Build history of the part. All positions in model axes, mm. Face numbers are marked on the shaded views. A direction names the side the tool comes from. Coordinates: 2 decimals unless noted, no trailing zeros. Loops run counter-clockwise (first coordinate to the right, second up) from the corner with the lowest first, then second, coordinate; pieces in that order, holes last.
(1) Slice it at D-D (y = 26). Give the cut face in (x, z), and give its area (3 significant figures).
(2) Wall check: L1, parallel to Y at x = 27.3, z = 8.5; L2, parallel to Y at x = 34, z = 25; L3, parallel to Y at x = 33.5, z = 10.5. Give the ranges that are in metal, low to high.
(3) Flat gauge pins, fed straight in: P1, Ø5, axis at x = 22.5, y = 15, coming from the +Z side; P2, Ø1, axis at x = 30, y = 16, coming from the -Z side; P3, Ø5, axis at y = 7, z = 4, coming from the -X side; P4, Ø4, axis at x = 45.7, z = 11.32, coming from the -Y side. Where does each tip first touch, or does it go through?
(4) Slice it at B-B (y = 2.5). Give the cut face in (x, z), and give its area (3 significant figures).
(5) Slice it at C-C (x = 25). Give the cut face in (y, z), and give its area (3 significant figures).
(6) Tool access for the marked faces 5, 6, 7 and 8: list every direction of +Z, -Z, +X, -X, +Y, -Y with a clear straight run to the whole face (end or side of a thin tool).
(7) Slice it at A-A (z = 17). Give the cut face in (x, y).
(8) Two-plate mould, pull along X, no slides. Class the marked faces 1, 2, 3 and 4: pulls with the +X half, pulls with the -X half, needs draft (parallel to the pull), parting line crosses it, or undercut.
from build123d import *

# Parameters (mm, degrees)
RESSALTO_EXTRUS_O1_DEPTH    = 30
CORTE_EXTRUS_O1_DEPTH       = 54.488316481
CORTE_EXTRUS_O1_DEPTH_BACK  = 54.488316481
ESBO_O3_R                   = 1.1
CORTE_EXTRUS_O6_DEPTH       = 54.488316481
CORTE_EXTRUS_O6_DEPTH_BACK  = 54.488316481
ESBO_O4_W                   = 12
ESBO_O4_H                   = 15
ESBO_O5_R                   = 1.6
CORTE_EXTRUS_O7_DEPTH       = 54.488316481
CORTE_EXTRUS_O9_START       = 6
ESBO_O7_W                   = 15
ESBO_O7_H                   = 15
CORTE_EXTRUS_O9_DEPTH       = 8
CORTE_EXTRUS_O11_REACH      = 55.488
ESBO_O9_R                   = 1.6
ESBO_O8_R                   = 3
CORTE_EXTRUS_O10_DEPTH      = 2
CORTE_EXTRUS_O14_DEPTH      = 43.308391603
CORTE_EXTRUS_O14_DEPTH_BACK = 2
CORTE_EXTRUS_O16_DEPTH      = 55.626001135
CORTE_EXTRUS_O16_DEPTH_BACK = 1
ESBO_O15_R                  = 2.1
FILETE1_R                   = 4
ESBO_O16_W                  = 10
ESBO_O16_H                  = 3.82
RESSALTO_EXTRUS_O2_DEPTH    = 2
ESBO_O17_W                  = 15.9
ESBO_O17_H                  = 2.8
RESSALTO_EXTRUS_O3_DEPTH    = 3.5
ESBO_O18_W                  = 52.248887689
ESBO_O18_H                  = 54.313207189
CORTE_EXTRUS_O17_DEPTH      = 34
ESBO_O19_R                  = 3.6
ESBO_O19_R_2                = 1.6
RESSALTO_EXTRUS_O4_DEPTH    = 6


with BuildPart() as part:
    # Esboço1 → Ressalto-extrusão1 (new body)
    with BuildSketch(Plane.XY):
        with BuildLine():
            Line((0, 0), (3, 0))
            Line((3, 0), (3, 8))
            ThreePointArc((3, 8), (4.464466094, 11.535533906), (8, 13))
            Line((8, 13), (15, 13))
            Line((15, 13), (15, 21))
            Line((15, 21), (-13, 21))
            Line((-13, 21), (-13, 36))
            Line((-13, 36), (1, 36))
            Line((1, 36), (1, 40))
            Line((1, 40), (-19, 40))
            Line((-19, 40), (-19, 17))
            Line((-19, 17), (0, 17))
            Line((0, 17), (0, 0))
        make_face()
    extrude(amount=RESSALTO_EXTRUS_O1_DEPTH)

    # Esboço3 → Corte-extrusão1 (cut, two sides: drawn at the far end of the back side and taken through both)
    with BuildSketch(Plane(origin=(0, 0, 0), x_dir=(0, 0, -1), z_dir=(1, 0, 0)).offset(-CORTE_EXTRUS_O1_DEPTH_BACK)):
        with Locations((-8.5, 14.5)):
            Circle(ESBO_O3_R)
        with Locations(Location((-21.5, 14.5, 0), (0, 0, 90))):
            Circle(ESBO_O3_R)
        with Locations(Location((-8.5, 2.5, 0), (0, 0, 90))):
            Circle(ESBO_O3_R)
        with Locations(Location((-21.5, 2.5, 0), (0, 0, 90))):
            Circle(ESBO_O3_R)
    extrude(amount=CORTE_EXTRUS_O1_DEPTH + CORTE_EXTRUS_O1_DEPTH_BACK, mode=Mode.SUBTRACT)

    # Esboço4 → Corte-extrusão6 (cut, two sides: drawn at the far end of the back side and taken through both)
    with BuildSketch(Plane(origin=(0, 0, 0), x_dir=(1, 0, 0), z_dir=(0, 1, 0)).offset(-CORTE_EXTRUS_O6_DEPTH_BACK)):
        with Locations((9, -22.5)):
            Rectangle(ESBO_O4_W, ESBO_O4_H)
    extrude(amount=CORTE_EXTRUS_O6_DEPTH + CORTE_EXTRUS_O6_DEPTH_BACK, mode=Mode.SUBTRACT)

    # Esboço5 → Corte-extrusão7 (cut, through all)
    with BuildSketch(Plane(origin=(0, 40, 0), x_dir=(1, 0, 0), z_dir=(0, 1, 0))):
        with Locations(Location((-5, -22, 0), (0, 0, 270))):
            Circle(ESBO_O5_R)
        with Locations(Location((-15.7, -11.32, 0), (0, 0, 180))):
            Circle(ESBO_O5_R)
        with Locations(Location((11, -7.5, 0), (0, 0, 180))):
            Circle(ESBO_O5_R)
    extrude(amount=-CORTE_EXTRUS_O7_DEPTH, mode=Mode.SUBTRACT)

    # Esboço7 → Corte-extrusão9 (cut)
    with BuildSketch(Plane(origin=(0, 21, 0), x_dir=(1, 0, 0), z_dir=(0, 1, 0)).offset(CORTE_EXTRUS_O9_START)):
        with Locations((-15.7, -11.32)):
            Rectangle(ESBO_O7_W, ESBO_O7_H)
    extrude(amount=CORTE_EXTRUS_O9_DEPTH, mode=Mode.SUBTRACT)

    # Esboço9 → Corte-extrusão11 (cut, up to next)
    with BuildSketch(Plane(origin=(0, 40, 0), x_dir=(1, 0, 0), z_dir=(0, 1, 0)), mode=Mode.PRIVATE) as corte_extrus_o11_sk1:
        with Locations(Location((-4, -7.5, 0), (0, 0, 180))):
            Circle(ESBO_O9_R)
    corte_extrus_o11_tool1 = extrude(corte_extrus_o11_sk1.sketch, amount=-CORTE_EXTRUS_O11_REACH, mode=Mode.PRIVATE) & part.part
    add(corte_extrus_o11_tool1.solids().sort_by_distance((-4, 40, 7.5))[0], mode=Mode.SUBTRACT)

    # Esboço8 → Corte-extrusão10 (cut)
    with BuildSketch(Plane(origin=(0, 40, 0), x_dir=(1, 0, 0), z_dir=(0, 1, 0))):
        with Locations(Location((-15.7, -11.32, 0), (0, 0, 180))):
            Circle(ESBO_O8_R)
        with Locations(Location((-5, -22, 0), (0, 0, 180))):
            Circle(ESBO_O8_R)
        with Locations(Location((-4, -7.5, 0), (0, 0, 180))):
            Circle(ESBO_O8_R)
    extrude(amount=-CORTE_EXTRUS_O10_DEPTH, mode=Mode.SUBTRACT)

    # Esboço14 → Corte-extrusão14 (cut, two sides: drawn at the far end of the back side and taken through both)
    with BuildSketch(Plane.XZ.offset(-17).offset(-CORTE_EXTRUS_O14_DEPTH_BACK)):
        with BuildLine():
            Line((11, 11), (15, 11))
            Line((15, 11), (15, 4))
            Line((15, 4), (11, 4))
            ThreePointArc((11, 4), (7.5, 7.5), (11, 11))
        make_face()
        Polygon((-5, 25.233161507), (-7.8, 23.616580754), (-7.8, 20.383419246), (-5, 18.766838493), (-2.2, 20.383419246), (-2.2, 23.616580754), align=None)
        Polygon((-15.7, 14.553161507), (-18.5, 12.936580754), (-18.5, 9.703419246), (-15.7, 8.086838493), (-12.9, 9.703419246), (-12.9, 12.936580754), align=None)
    extrude(amount=CORTE_EXTRUS_O14_DEPTH + CORTE_EXTRUS_O14_DEPTH_BACK, mode=Mode.SUBTRACT)

    # Esboço15 → Corte-extrusão16 (cut, two sides: drawn at the far end of the back side and taken through both)
    with BuildSketch(Plane(origin=(3, 0, 0), x_dir=(0, 0, -1), z_dir=(1, 0, 0)).offset(-CORTE_EXTRUS_O16_DEPTH_BACK)):
        with Locations(Location((-21.5, 14.5, 0), (0, 0, 90))):
            Circle(ESBO_O15_R)
        with Locations(Location((-8.5, 14.5, 0), (0, 0, 313.540252108))):
            Circle(ESBO_O15_R)
        with Locations(Location((-8.5, 2.5, 0), (0, 0, 90))):
            Circle(ESBO_O15_R)
        with Locations(Location((-21.5, 2.5, 0), (0, 0, 90))):
            Circle(ESBO_O15_R)
    extrude(amount=CORTE_EXTRUS_O16_DEPTH + CORTE_EXTRUS_O16_DEPTH_BACK, mode=Mode.SUBTRACT)

    # Filete1
    # the kernel refuses this fillet: 4 mm, written as the material it adds along each edge
    with BuildSketch(Plane(origin=(-13, 21, 0), x_dir=(1, 0, 0), z_dir=(0, 0, 1))) as filete1_piece_1:
        with BuildLine():
            CenterArc((FILETE1_R, FILETE1_R), FILETE1_R, 180, 90)
            Line((0, FILETE1_R), (0, 0))
            Line((0, 0), (FILETE1_R, 0))
        make_face()
    extrude(amount=30)
    with BuildSketch(Plane(origin=(-13, 36, 0), x_dir=(1, 0, 0), z_dir=(0, 0, 1))) as filete1_piece_2_section:
        with BuildLine():
            CenterArc((FILETE1_R, -FILETE1_R), FILETE1_R, 90, 90)
            Line((0, -FILETE1_R), (0, 0))
            Line((0, 0), (FILETE1_R, 0))
        make_face()
    filete1_piece_2 = extrude(amount=30, mode=Mode.PRIVATE)
    filete1_piece_2 = split(filete1_piece_2, bisect_by=Plane(origin=(-11.759467995, 35, 1.91), z_dir=(0, 1, 0)), keep=Keep.TOP, mode=Mode.PRIVATE)
    filete1_piece_2 = split(filete1_piece_2, bisect_by=Plane(origin=(-11.759467995, 35.634662641, 3.82), z_dir=(0, 0, -1)), keep=Keep.TOP, mode=Mode.PRIVATE)
    add(filete1_piece_2)
    with BuildSketch(Plane(origin=(-13, 36, 0), x_dir=(1, 0, 0), z_dir=(0, 0, 1))) as filete1_piece_3_section:
        with BuildLine():
            CenterArc((FILETE1_R, -FILETE1_R), FILETE1_R, 90, 90)
            Line((0, -FILETE1_R), (0, 0))
            Line((0, 0), (FILETE1_R, 0))
        make_face()
    filete1_piece_3 = extrude(amount=30, mode=Mode.PRIVATE)
    filete1_piece_3 = split(filete1_piece_3, bisect_by=Plane(origin=(-12.678584174, 35, 1.91), z_dir=(0, -1, 0)), keep=Keep.TOP, mode=Mode.PRIVATE)
    filete1_piece_3 = split(filete1_piece_3, bisect_by=Plane(origin=(-12.678584174, 34.15222085, 3.82), z_dir=(0, 0, -1)), keep=Keep.TOP, mode=Mode.PRIVATE)
    add(filete1_piece_3)
    with BuildSketch(Plane(origin=(-13, 36, 0), x_dir=(1, 0, 0), z_dir=(0, 0, 1))) as filete1_piece_4_section:
        with BuildLine():
            CenterArc((FILETE1_R, -FILETE1_R), FILETE1_R, 90, 90)
            Line((0, -FILETE1_R), (0, 0))
            Line((0, 0), (FILETE1_R, 0))
        make_face()
    filete1_piece_4 = extrude(amount=30, mode=Mode.PRIVATE)
    filete1_piece_4 = split(filete1_piece_4, bisect_by=Plane(origin=(-11.759467995, 35, 11.32), z_dir=(0, 1, 0)), keep=Keep.TOP, mode=Mode.PRIVATE)
    filete1_piece_4 = split(filete1_piece_4, bisect_by=Plane(origin=(-11.759467995, 35.634662641, 3.82), z_dir=(0, 0, 1)), keep=Keep.TOP, mode=Mode.PRIVATE)
    filete1_piece_4 = split(filete1_piece_4, bisect_by=Plane(origin=(-11.759467995, 35.634662641, 18.82), z_dir=(0, 0, -1)), keep=Keep.TOP, mode=Mode.PRIVATE)
    add(filete1_piece_4)
    with BuildSketch(Plane(origin=(-13, 36, 0), x_dir=(1, 0, 0), z_dir=(0, 0, 1))) as filete1_piece_5_section:
        with BuildLine():
            CenterArc((FILETE1_R, -FILETE1_R), FILETE1_R, 90, 90)
            Line((0, -FILETE1_R), (0, 0))
            Line((0, 0), (FILETE1_R, 0))
        make_face()
    filete1_piece_5 = extrude(amount=30, mode=Mode.PRIVATE)
    filete1_piece_5 = split(filete1_piece_5, bisect_by=Plane(origin=(-11.759467995, 35, 24.41), z_dir=(0, 1, 0)), keep=Keep.TOP, mode=Mode.PRIVATE)
    filete1_piece_5 = split(filete1_piece_5, bisect_by=Plane(origin=(-11.759467995, 35.634662641, 18.82), z_dir=(0, 0, 1)), keep=Keep.TOP, mode=Mode.PRIVATE)
    add(filete1_piece_5)
    with BuildSketch(Plane(origin=(-13, 36, 0), x_dir=(1, 0, 0), z_dir=(0, 0, 1))) as filete1_piece_6_section:
        with BuildLine():
            CenterArc((FILETE1_R, -FILETE1_R), FILETE1_R, 90, 90)
            Line((0, -FILETE1_R), (0, 0))
            Line((0, 0), (FILETE1_R, 0))
        make_face()
    filete1_piece_6 = extrude(amount=30, mode=Mode.PRIVATE)
    filete1_piece_6 = split(filete1_piece_6, bisect_by=Plane(origin=(-12.678584174, 35, 24.41), z_dir=(0, -1, 0)), keep=Keep.TOP, mode=Mode.PRIVATE)
    filete1_piece_6 = split(filete1_piece_6, bisect_by=Plane(origin=(-12.678584174, 34.15222085, 18.82), z_dir=(0, 0, 1)), keep=Keep.TOP, mode=Mode.PRIVATE)
    add(filete1_piece_6)
    # the kernel refuses this fillet: 4 mm, written as the material it takes off along each edge
    with BuildSketch(Plane(origin=(-10, 0, 0), x_dir=(0, 0, 1), z_dir=(1, 0, 0))) as filete1_2_piece_1:
        with BuildLine():
            CenterArc((FILETE1_R, -FILETE1_R), FILETE1_R, 90, 90)
            Line((0, -FILETE1_R), (0, 0))
            Line((0, 0), (FILETE1_R, 0))
        make_face()
    extrude(amount=23, mode=Mode.SUBTRACT)
    with BuildSketch(Plane(origin=(-10, 0, 30), x_dir=(0, 0, -1), z_dir=(1, 0, 0))) as filete1_2_piece_2:
        with BuildLine():
            CenterArc((FILETE1_R, FILETE1_R), FILETE1_R, 180, 90)
            Line((0, FILETE1_R), (0, 0))
            Line((0, 0), (FILETE1_R, 0))
        make_face()
    extrude(amount=23, mode=Mode.SUBTRACT)
    with BuildSketch(Plane(origin=(3, 21, 15), x_dir=(-1, 0, 0), z_dir=(0, 0, 1))) as filete1_2_piece_3:
        with BuildLine():
            CenterArc((FILETE1_R, FILETE1_R), FILETE1_R, 180, 90)
            Line((0, FILETE1_R), (0, 0))
            Line((0, 0), (FILETE1_R, 0))
        make_face()
    extrude(amount=25, mode=Mode.SUBTRACT)
    with BuildSketch(Plane(origin=(1, 26, 0), x_dir=(0, 0, 1), z_dir=(0, 1, 0)), Plane(origin=(15, 13, -10), x_dir=(-1, 0, 0), z_dir=(0, 0, 1)), Plane(origin=(15, 13, 1), x_dir=(-1, 0, 0), z_dir=(0, 0, 1))) as filete1_2_piece_4:
        with BuildLine():
            CenterArc((FILETE1_R, -FILETE1_R), FILETE1_R, 90, 90)
            Line((0, -FILETE1_R), (0, 0))
            Line((0, 0), (FILETE1_R, 0))
        make_face()
    extrude(amount=24, mode=Mode.SUBTRACT)
    with BuildSketch(Plane(origin=(1, 26, 30), x_dir=(0, 0, -1), z_dir=(0, 1, 0))) as filete1_2_piece_5:
        with BuildLine():
            CenterArc((FILETE1_R, FILETE1_R), FILETE1_R, 180, 90)
            Line((0, FILETE1_R), (0, 0))
            Line((0, 0), (FILETE1_R, 0))
        make_face()
    extrude(amount=24, mode=Mode.SUBTRACT)

    # Esboço16 → Ressalto-extrusão2 (add)
    with BuildSketch(Plane(origin=(0, 21, 0), x_dir=(1, 0, 0), z_dir=(0, 1, 0))):
        with Locations((-14, -1.91)):
            Rectangle(ESBO_O16_W, ESBO_O16_H)
    extrude(amount=RESSALTO_EXTRUS_O2_DEPTH)

    # Esboço17 → Ressalto-extrusão3 (add)
    with BuildSketch(Plane(origin=(0, 21, 0), x_dir=(1, 0, 0), z_dir=(0, 1, 0))):
        with Locations((-1.05, -7.5)):
            Rectangle(ESBO_O17_W, ESBO_O17_H)
    extrude(amount=RESSALTO_EXTRUS_O3_DEPTH)

    # Espelhar1: part across plane


with BuildPart() as part_1:
    add(part.part)
    add(part.part.mirror(Plane(origin=(15, 21, 30), x_dir=(0, 0, 1), z_dir=(-1, 0, 0))))

    # Esboço18 → Corte-extrusão17 (cut)
    with BuildSketch(Plane.ZY.offset(19)):
        with Locations((14.699236255, 19.293263453)):
            Rectangle(ESBO_O18_W, ESBO_O18_H)
    extrude(amount=-CORTE_EXTRUS_O17_DEPTH, mode=Mode.SUBTRACT)

    # Esboço19 → Ressalto-extrusão4 (add)
    with BuildSketch(Plane.XZ.offset(-36)):
        with Locations(Location((35, 22, 0), (0, 0, 180))):
            Circle(ESBO_O19_R)
        with Locations(Location((35, 22, 0), (0, 0, 270))):
            Circle(ESBO_O19_R_2, mode=Mode.SUBTRACT)
    extrude(amount=RESSALTO_EXTRUS_O4_DEPTH)


solid = part_1.part
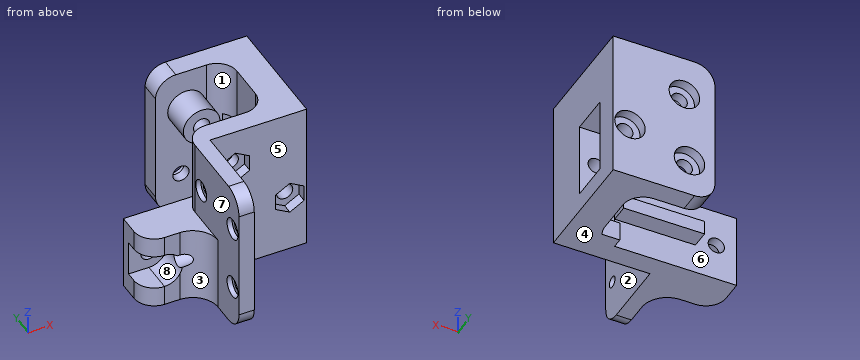
Response values:
1. outline: (43, 0) - (49, 0) - (49, 30) - (43, 30) - close; hole circle Ø3.2 at (45.7, 11.32)
1. area: 172 mm2
2. L1: y = 0 to 0.4, 4.6 to 12.4, 16.6 to 24.5
2. L2: y = 17 to 21, 30 to 40
2. L3: y = 17 to 21, 36 to 40
3. P1: stops at z = 15
3. P2: stops at z = 0
3. P3: stops at x = 26.77
3. P4: stops at y = 19
4. outline: (27, 0.29) - (30, 0.29) - (30, 7.4) - (28, 7.4) - (28, 6.4) - (27, 6.4) - close; (27, 10.6) - (28, 10.6) - (28, 9.6) - (30, 9.6) - (30, 20.4) - (28, 20.4) - (28, 19.4) - (27, 19.4) - close; (27, 23.6) - (28, 23.6) - (28, 22.6) - (30, 22.6) - (30, 29.71) - (27, 29.71) - close
4. area: 71.0 mm2
5. outline: (12, 0) - (21, 0) - (21, 6.1) - (24.5, 6.1) - (24.5, 8.9) - (21, 8.9) - (21, 15) - (12, 15) - close; hole circle Ø4.2 at (14.5, 8.5)
5. area: 131 mm2
6. face 5: +Z, -Z, +X, -Y
6. face 6: -X
6. face 7: +Z, -X, -Y
6. face 8: -X, -Y
7. outline: (27, 0) - (30, 0) - (30, 17) - (49, 17) - (49, 27) - (43, 27) - (43, 25) arc R4 cw to (39, 21) - (31, 21) arc R4 ccw to (27, 17) - close; (29, 36) - (39, 36) arc R4 cw to (41.65, 35) - (49, 35) - (49, 40) - (29, 40) - close
8. face 1: undercut
8. face 2: pulls with the +X half
8. face 3: pulls with the -X half
8. face 4: needs draft
